```python
from build123d import *

# Parameters (mm, degrees)
F0_W     = 20
F0_H     = 20
F1_DEPTH = 6
F2_W     = 6.5
F2_H     = 5.5
F3_DEPTH = 3
F4_R     = 2.75
F5_DEPTH = 9.001


with BuildPart() as f1:
    # F0 (on Top) → F1 (new body)
    with BuildSketch(Plane.XY):
        Rectangle(F0_W, F0_H)
    extrude(amount=F1_DEPTH)

    # F2 (on face) → F3 (join)
    with BuildSketch(Plane.XY.offset(6)):
        with Locations((6.75, 0)):
            Rectangle(F2_W, F2_H)
        with Locations((-6.75, 0)):
            Rectangle(F2_W, F2_H)
    extrude(amount=F3_DEPTH)

    # F4 (on face) → F5 (cut, through all)
    with BuildSketch(Plane(origin=(0, 0, 0), x_dir=(1, 0, 0), z_dir=(0, 0, -1))):
        Circle(F4_R)
    extrude(amount=-F5_DEPTH, mode=Mode.SUBTRACT)


solid = f1.part
```
Input: part model. Units: mm. Frame: model coordinates. A direction names the side the tool comes from. Give positions to 0.01 mm unless a question says otherwise; leave off trailing zeros. Order: outer loops, then holes, each group sorted by start corner. A loop starts at its lowest first (then second) coordinate and runs counter-clockwise, first axis right, second up.
1. Section B-B on y = 0. Return the cut outline in (x, z), and give its area (3 significant figures).
Derived:
outline: (-10, 0) - (-2.75, 0) - (-2.75, 6) - (-3.5, 6) - (-3.5, 9) - (-10, 9) - close; (2.75, 0) - (10, 0) - (10, 9) - (3.5, 9) - (3.5, 6) - (2.75, 6) - close
area: 126 mm2
2. Material intervals for L1, parallel to Y at x = 0, z = 1.7; L2, parallel to Z at x = 0.5, y = -7.25, sorted ascending.
Derived:
L1: y = -10 to -2.75, 2.75 to 10
L2: z = 0 to 6
3. Section A-A on z = 8. Return the cut outline in (x, y).
Derived:
outline: (-10, -2.75) - (-3.5, -2.75) - (-3.5, 2.75) - (-10, 2.75) - close; (3.5, -2.75) - (10, -2.75) - (10, 2.75) - (3.5, 2.75) - close
4. Section C-C on x = 0. Return the cut outline in (y, z), and give its area (3 significant figures).
Derived:
outline: (-10, 0) - (-2.75, 0) - (-2.75, 6) - (-10, 6) - close; (2.75, 0) - (10, 0) - (10, 6) - (2.75, 6) - close
area: 87.0 mm2
5. Section D-D on z = 3.75. Return the cut outline in (x, y), and give its area (3 significant figures).
Derived:
outline: (-10, -10) - (10, -10) - (10, 10) - (-10, 10) - close; hole circle Ø5.5 at (0, 0)
area: 376 mm2
6. Reachability of faces 5 (the flat face through (0, -10, 3)), 6 (the flat face through (-7, 2.75, 7)), 7 (the flat face through (-7, -2.75, 7)) from +Z, -Z, +X, -X, +Y, -Y: full face, straight path, thin tool, end or side. Return the list, or none.
Derived:
face 5: +Z, -Z, +X, -X, -Y
face 6: +Z, +X, -X, +Y
face 7: +Z, +X, -X, -Y
7. Mould query, pull axis X, two halves, no side actions, for faces 1 (the flat face through (0, 10, 3)), 2 (the flat face through (-3.5, 0, 7)), 3 (the flat face through (3.5, 0, 7)), 4 (the flat face through (10, 0, 3)). Classes: released by +X, released by -X, zero draft, split by the parting line, or undercut.
Derived:
face 1: zero draft
face 2: undercut
face 3: undercut
face 4: released by +X
8. Pin query (flat end, axial travel): pin 1 (2.5 mm diameter, centred on x = 6.5, z = 7.5, fed in from +Y); pin 2 (1.5 mm diameter, centred on x = -5.5, z = 7.5, fed in from -Y); pin 3 (5 mm diameter, centred on x = 0, y = 0, fed in from +Z). Return the tip coordinate at first contact, or that it passes through.
Derived:
pin 1: stops at y = 2.75
pin 2: stops at y = -2.75
pin 3: passes through
